Design review of the part shown in the three views and the two pictorial views. Dimensions are in mm from the part's minimum x, y and z. A direction names the side the tool comes from. Give positions to 0.01 mm unless a question says otherwise; leave off trailing zeros. Loops run counter-clockwise (first coordinate to the right, second up) from the corner with the lowest first, then second, coordinate; pieces in that order, holes last. Notation, with made-up numbers: (60.25, 37) -> (99.25, 37) arc R10 ccw to (99.25, 53) -> close; hole circle Ø1 at (41.25, -5). An arc over 180 degrees is marked (long way). Use CSV: the item, a comma, the result in double quotes. Start each with the question number.
Item 1: For the marked faces 1 and 2, list the 3-axis set-ups (+Z, -Z, +X, -X, +Y, -Y) from which the entire face can be reached by the end or side of a thin tool; tool diameter is ignored.
Item 2: We need section B-B (z = 9.25). State the section outline as (x, y) points, plus the area to 3 significant figures.
Item 3: Clearance check with flat-ended pins moving along their axes: pin 1 (1.5 mm diameter, centred on x = 4.5, y = 5, fed in from +Z); pin 2 (5 mm diameter, centred on y = 14.5, z = 7.5, fed in from -X); pin 3 (2 mm diameter, centred on x = 2, y = 6.5, fed in from +Z). State where each tip first meets the part, or that it passes through.
Item 4: Wall thickness on line 1 along Y through (x, z) = (1.75, 8); line 2 along Z through (x, y) = (3.5, 13.25); line 3 along Y through (x, z) = (6.25, 9): over which ranges is each line inside the solid? List them lowest first. Write a range as from..to.
Item 5: We need section C-C (x = 5). State the section outline as (y, z) points, plus the area to 3 significant figures.
Item 6: The part is to be moulded in two halves that separate along Y. For the marked faces 3, 4, 5 and 6, say which applies: +Y half, -Y half, draft (parallel to the pull), parting line (faces both ways), or undercut.
Item 7: We need section D-D (z = 5). State the section outline as (x, y) points.
Item 8: We need section A-A (y = 2). State the section outline as (x, z) points.
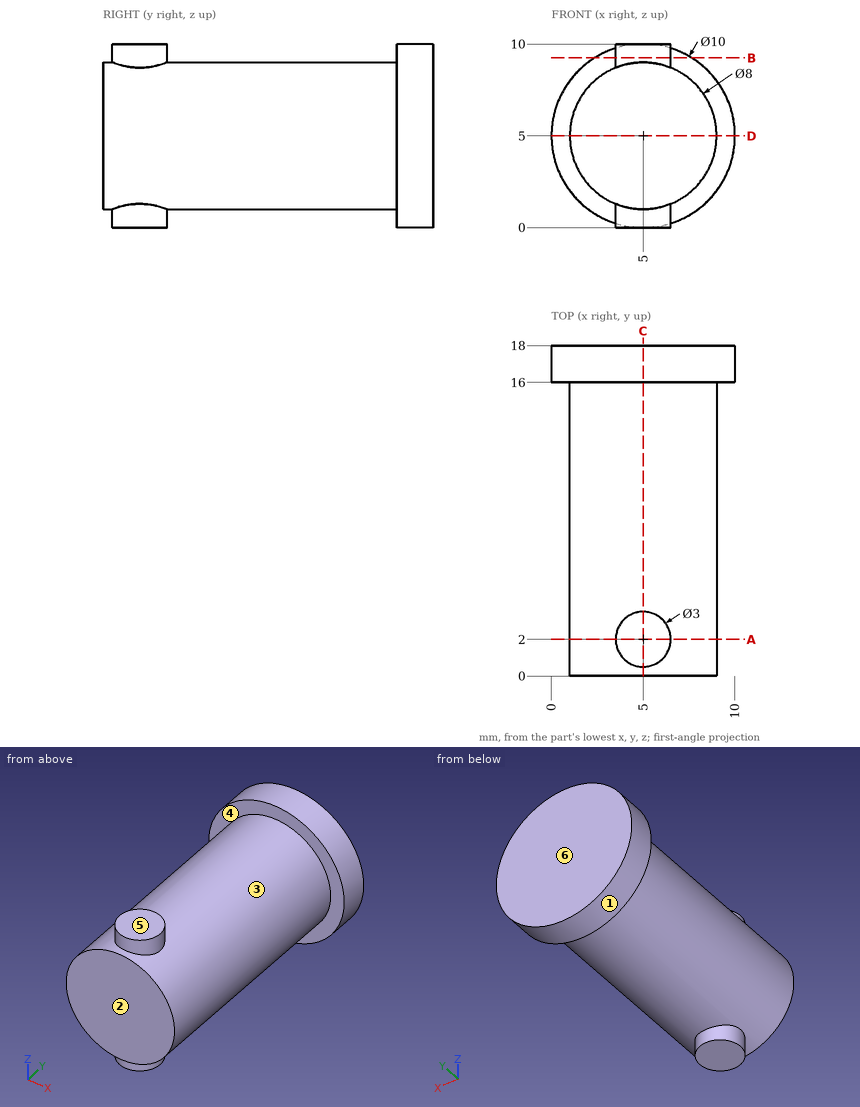
Results found:
1,face 1,"+Y"
1,face 2,"+Z, -Z, +X, -X, -Y"
2,outline,"(2.37, 16) -> (7.63, 16) -> (7.63, 18) -> (2.37, 18) -> close; circle Ø3 at (5, 2)"
2,area,"17.6 mm²"
3,pin 1,"z = 9"
3,pin 2,"x = 0.03"
3,pin 3,"z = 8.46"
4,line 1,"16..18"
4,line 2,"1.29..8.71"
4,line 3,"1.17..2.83, 16..18"
5,outline,"(0, 1) -> (0.5, 1) -> (0.5, 0) -> (3.5, 0) -> (3.5, 1) -> (16, 1) -> (16, 0) -> (18, 0) -> (18, 10) -> (16, 10) -> (16, 9) -> (3.5, 9) -> (3.5, 10) -> (0.5, 10) -> (0.5, 9) -> (0, 9) -> close"
5,area,"154 mm²"
6,face 3,"undercut"
6,face 4,"undercut"
6,face 5,"draft"
6,face 6,"+Y half"
7,outline,"(0, 16) -> (1, 16) -> (1, 0) -> (9, 0) -> (9, 16) -> (10, 16) -> (10, 18) -> (0, 18) -> close"
8,outline,"(3.5, 0) -> (6.5, 0) -> (6.5, 1.29) arc R4 ccw to (6.5, 8.71) -> (6.5, 10) -> (3.5, 10) -> (3.5, 8.71) arc R4 ccw to (3.5, 1.29) -> close"
